Design review of the part shown in the three views and the two pictorial views. Dimensions are in mm from the part's minimum x, y and z. A direction names the side the tool comes from. Round coordinates to 2 decimals unless told otherwise and drop trailing zeros. Write each loop counter-clockwise with the first axis right and the second up, starting at its lowest first coordinate (ties: lowest second). Pieces come first, ordered by that corner, then holes. Notation, with made-up numbers: (20.5, 31.25) -> (62.5, 31.25) arc R16 ccw to (62.5, 49.25) -> close; hole circle Ø9 at (87.25, -7). An arc over 180 degrees is marked (long way). Answer as a JSON object with one key per item and string values. Group by question number.
1) We need section B-B, the plane y = 43. Count the separate pieces of the cut face and the enclosed holes in it, then the cut area to 3 significant figures.
2) Insertion check: pin 1 Ø1.5 at (y, z) = (36, 60.5) entering from +X (1 decimal); pin 2 Ø8 at (y, z) = (28.5, 68) entering from -X (1 decimal); pin 3 Ø4 at (y, z) = (31.5, 22) entering from -X. Each pin has a flat end and moves straight along its axis. Give the tip position at first contact, or say it passes through.
3) Mouldability with a two-part tool opening along X and no side actions: class the marked faces 1, 2, 3 and 4 as pulls with the +X half, pulls with the -X half, needs draft (parallel to the pull), parting line crosses it, or undercut.
4) We need section A-A, the plane x = 56. Write out the cut boundary in (y, z) (1 decimal), then the cut area to 3 significant figures.
5) We need section C-C, the plane x = 90. Write out the cut boundary in (y, z), then the cut area to 3 significant figures.
6) Machinability: for the marked faces 5 and 6, which of the approach directions +Z, -Z, +X, -X, +Y, -Y give a long, thin tool a straight path to every point of the face, cutting with its end or side? Answer none if there is none.
7) To check wall thickness, follow probe 1 along Z at (x, y) = (105, 43); probe 2 along Y at (x, z) = (97.5, 34.5); probe 3 along X at (y, z) = (24, 36.5) (1 decimal). State the ranges of each line that lie inside material, in increasing order. Write a range as [from, to].
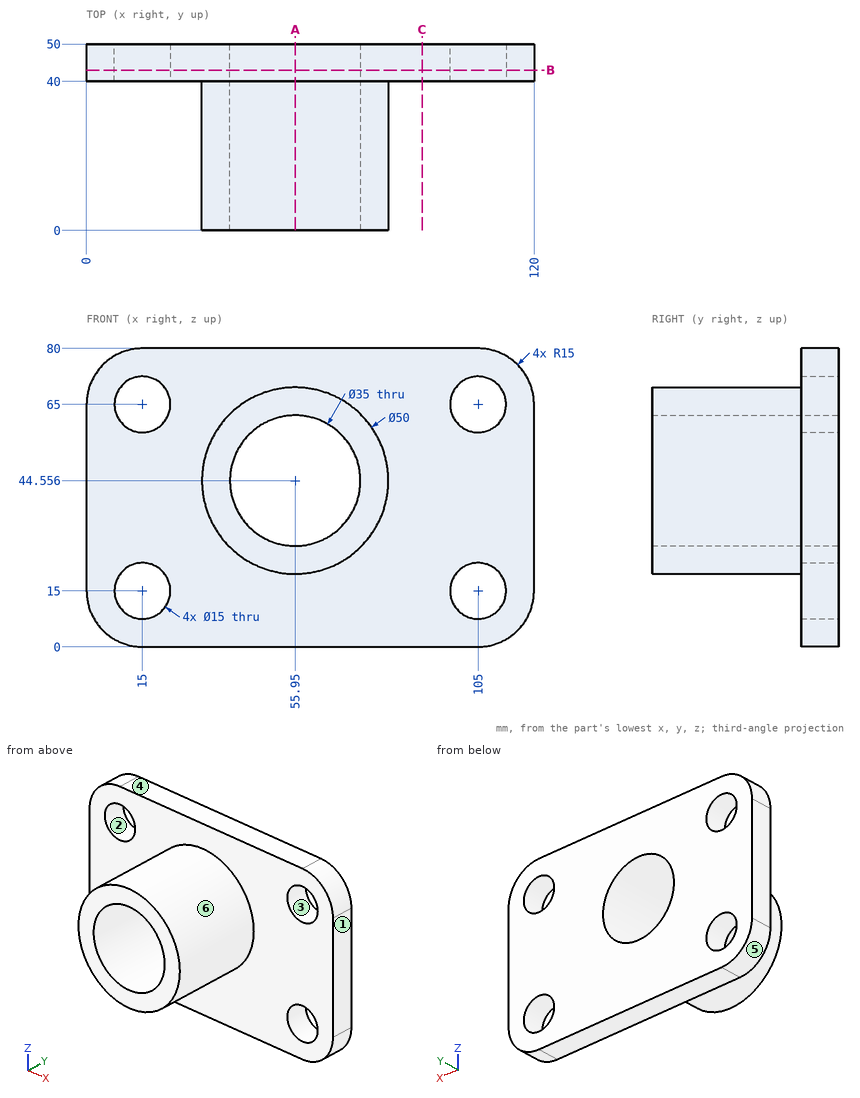
Here are the results:
{
 "1": {"separate pieces": "1", "enclosed holes": "5", "area": "7,740 mm^2"},
 "2": {"pin 1": "stops at x = 75.8", "pin 2": "stops at x = 40.2", "pin 3": "stops at x = 41.72"},
 "3": {"face 1": "pulls with the +X half", "face 2": "undercut", "face 3": "undercut", "face 4": "needs draft"},
 "4": {"outline": "(0, 19.6) -> (40, 19.6) -> (40, 0) -> (50, 0) -> (50, 27.1) -> (0, 27.1) -> close; (0, 62.1) -> (50, 62.1) -> (50, 80) -> (40, 80) -> (40, 69.6) -> (0, 69.6) -> close", "area": "1,050 mm^2"},
 "5": {"outline": "(40, 0) -> (50, 0) -> (50, 80) -> (40, 80) -> close", "area": "800 mm^2"},
 "6": {"face 5": "-Z, -X, +Y, -Y", "face 6": "-Y"},
 "7": {"probe 1": "z = [0, 7.5], [22.5, 57.5], [72.5, 80]", "probe 2": "y = [40, 50]", "probe 3": "x = [32.3, 40.4], [71.5, 79.6]"}
}
